from build123d import *

# Parameters (mm, degrees)
BOSS_EXTRUDE2_DEPTH = 12
SKETCH2_W           = 12
SKETCH2_H           = 22.5
BOSS_EXTRUDE3_DEPTH = 6
SKETCH3_W           = 12
SKETCH3_H           = 22.5
BOSS_EXTRUDE4_DEPTH = 6
SKETCH4_R           = 1.75
CUT_EXTRUDE1_DEPTH  = 22.5
FILLET1_R           = 2
BOSS_EXTRUDE5_START = 4.65
BOSS_EXTRUDE5_DEPTH = 4.65
SKETCH6_W           = 26.4
SKETCH6_H           = 18
SKETCH6_R           = 4.925
BOSS_EXTRUDE6_DEPTH = 2.5


with BuildPart() as part:
    # Sketch1 → Boss-Extrude2 (new body)
    with BuildSketch(Plane.XY):
        Polygon((0, 18), (0, 0), (17.3, 0), (17.3, 7.6), (17.3, 15.2), (20.697059459, 15.2), (34.302940541, 15.2), (37.7, 15.2), (37.7, 7.6), (37.7, 0), (55, 0), (55, 18), align=None)
        with BuildLine():
            Line((17.3, 15.2), (17.3, 7.6))
            ThreePointArc((17.3, 7.6), (18.187911257, 11.762331467), (20.697059459, 15.2))
            Line((20.697059459, 15.2), (17.3, 15.2))
        make_face()
        with BuildLine():
            Line((37.7, 15.2), (34.302940541, 15.2))
            ThreePointArc((34.302940541, 15.2), (36.812088743, 11.762331467), (37.7, 7.6))
            Line((37.7, 7.6), (37.7, 15.2))
        make_face()
    extrude(amount=BOSS_EXTRUDE2_DEPTH)

    # Sketch2 → Boss-Extrude3 (add)
    with BuildSketch(Plane.ZY):
        with Locations((6, 6.75)):
            Rectangle(SKETCH2_W, SKETCH2_H)
    extrude(amount=BOSS_EXTRUDE3_DEPTH)

    # Sketch3 → Boss-Extrude4 (add)
    with BuildSketch(Plane(origin=(55, 0, 0), x_dir=(0, 0, -1), z_dir=(1, 0, 0))):
        with Locations((-6, 6.75)):
            Rectangle(SKETCH3_W, SKETCH3_H)
    extrude(amount=BOSS_EXTRUDE4_DEPTH)

    # Sketch4 → Cut-Extrude1 (cut)
    with BuildSketch(Plane(origin=(0, 18, 0), x_dir=(1, 0, 0), z_dir=(0, 1, 0))):
        with Locations(Location((-3, -7, 0), (0, 0, 270))):
            Circle(SKETCH4_R)
        with Locations(Location((58, -7, 0), (0, 0, 270))):
            Circle(SKETCH4_R)
    extrude(amount=-CUT_EXTRUDE1_DEPTH, mode=Mode.SUBTRACT)

    # Fillet1
    # the kernel refuses this fillet: 2 mm, written as the material it takes off along each edge
    with BuildSketch(Plane(origin=(-3, 18, 7), x_dir=(0, 0, 1), z_dir=(-1, 0, 0))) as fillet1_piece_1:
        with BuildLine():
            CenterArc((1.75 + FILLET1_R, -FILLET1_R), FILLET1_R, 90, 90)
            Line((1.75, -FILLET1_R), (1.75, 0))
            Line((1.75, 0), (1.75 + FILLET1_R, 0))
        make_face()
    revolve(axis=Axis((-3, 18, 7), (0, 1, 0)), mode=Mode.SUBTRACT)
    with BuildSketch(Plane(origin=(58, 18, 7), x_dir=(0, 0, 1), z_dir=(-1, 0, 0))) as fillet1_piece_2:
        with BuildLine():
            CenterArc((1.75 + FILLET1_R, -FILLET1_R), FILLET1_R, 90, 90)
            Line((1.75, -FILLET1_R), (1.75, 0))
            Line((1.75, 0), (1.75 + FILLET1_R, 0))
        make_face()
    revolve(axis=Axis((58, 18, 7), (0, 1, 0)), mode=Mode.SUBTRACT)

    # Sketch5 → Boss-Extrude5 (add)
    with BuildSketch(Plane(origin=(0, 0, 0), x_dir=(-1, 0, 0), z_dir=(0, 0, -1)).offset(BOSS_EXTRUDE5_START)):
        with BuildLine():
            Line((-37.7, 0), (-40.7, 0))
            Line((-40.7, 0), (-40.7, 18))
            Line((-40.7, 18), (-14.3, 18))
            Line((-14.3, 18), (-14.3, 0))
            Line((-14.3, 0), (-17.3, 0))
            Line((-17.3, 0), (-17.3, 6))
            ThreePointArc((-17.3, 6), (-18.898767331, 7.537206525), (-17.425490196, 9.195071224))
            ThreePointArc((-17.425490196, 9.195071224), (-18.543054375, 12.47986937), (-20.697059459, 15.2))
            Line((-20.697059459, 15.2), (-34.302940541, 15.2))
            ThreePointArc((-34.302940541, 15.2), (-36.456945625, 12.47986937), (-37.574509804, 9.195071224))
            ThreePointArc((-37.574509804, 9.195071224), (-36.101232669, 7.537206525), (-37.7, 6))
            Line((-37.7, 6), (-37.7, 0))
        make_face()
    extrude(amount=-BOSS_EXTRUDE5_DEPTH)

    # Sketch6 → Boss-Extrude6 (add)
    with BuildSketch(Plane(origin=(0, 0, -4.65), x_dir=(-1, 0, 0), z_dir=(0, 0, -1))):
        with Locations((-27.5, 9)):
            Rectangle(SKETCH6_W, SKETCH6_H)
        with Locations((-27.5, 7.537206525)):
            Circle(SKETCH6_R, mode=Mode.SUBTRACT)
    extrude(amount=BOSS_EXTRUDE6_DEPTH)


solid = part.part
Verification items for the finished model (mm, model axes). A direction names the side the tool comes from. Give positions to 0.01 mm unless a question says otherwise; leave off trailing zeros. Order: outer loops, then holes, each group sorted by start corner. A loop starts at its lowest first (then second) coordinate and runs counter-clockwise, first axis right, second up. Notation, with made-up numbers: M 13,32.5 L 25,32.5 A15 ccw 25,61.5 Z; hole C 28.5,57 d10. An arc over 180 degrees is marked long. Use one line per item in the form item = value. Start each with the question number.
Q1. Mould release check, pull along Y, two halves, no side actions. Record for faces 1 (the cylindrical face through (36.1, 7.6, -2.4)), 2 (the flat face through (55, -2, 6)), 3 (the flat face through (28, 18, 5)), 4 (the cylindrical face through (31.41, 4.54, -5.88)): +Y half, -Y half, draft (parallel to the pull), parting line (faces both ways), or undercut.
Q2. Scan lines: line 1 along X through (y, z) = (2.5, 7); line 2 along X through (y, z) = (-1.5, 1.5); line 3 along Y through (x, z) = (27.5, -5.7). Record each from-to range of solid material in increasing order. Write a range as [from, to].
Q3. Section check B-B (y = 1.5). Enter the section's corners in (x, z).
Q4. Go/stop test with flat-tipped pins: pin 1 Ø8 at (x, y) = (27, -0.5) entering from +Z; pin 2 Ø6 at (x, y) = (7, 6.5) entering from -Z; pin 3 Ø1 at (y, z) = (5.5, -1) entering from +X. Record where each tip stops, or that it passes through.
Q5. Section check C-C (z = 7). Enter the section's corners in (x, y), then the cut area to 3 significant figures.
Q6. Section check A-A (x = -3). Enter the section's corners in (y, z).
Q7. Section check D-D (y = 11.5). Enter the section's corners in (x, z).
Q8. Access from +Z, -Z, +X, -X, +Y, -Y to the whole of each face (thin tool, end or side, straight path). Record for faces 5 (the flat face through (51, 9, 0)), 6 (the flat face through (17.3, 4, 4)), 7 (the flat face through (28, 0, -6)).
Evaluation:
q1.face_1 = undercut
q1.face_2 = draft
q1.face_3 = +Y half
q1.face_4 = undercut
q2.line_1 = [-6, -4.75], [-1.25, 17.3], [37.7, 56.25], [59.75, 61]
q2.line_2 = [-6, 0], [55, 61]
q2.line_3 = [0, 2.61], [12.46, 18]
q3.outline = M -6,0 L 14.3,0 L 14.3,-7.15 L 40.7,-7.15 L 40.7,0 L 61,0 L 61,12 L 37.7,12 L 37.7,-4.65 L 17.3,-4.65 L 17.3,12 L -6,12 Z; hole C -3,7 d3.5; hole C 58,7 d3.5
q4.pin_1 = -4.65
q4.pin_2 = 0
q4.pin_3 = 40.7
q5.outline = M -6,-4.5 L -4.75,-4.5 L -4.75,16 A2 ccw -6,17.85 Z; M -1.25,-4.5 L 0,-4.5 L 0,0 L 17.3,0 L 17.3,7.6 A10.2 cw 20.7,15.2 L 34.3,15.2 A10.2 cw 37.7,7.6 L 37.7,0 L 55,0 L 55,-4.5 L 56.25,-4.5 L 56.25,16 A2 ccw 54.25,18 L 0.75,18 A2 ccw -1.25,16 Z; M 59.75,-4.5 L 61,-4.5 L 61,17.85 A2 ccw 59.75,16 Z
q5.area = 805 mm2
q6.outline = M -4.5,0 L 18,0 L 18,3.25 A2 ccw 16,5.25 L -4.5,5.25 Z; M -4.5,8.75 L 16,8.75 A2 ccw 18,10.75 L 18,12 L -4.5,12 Z
q7.outline = M -6,0 L 14.3,0 L 14.3,-7.15 L 24.58,-7.15 L 24.58,-4.65 L 18.08,-4.65 L 18.08,12 L -6,12 Z; M 30.42,-7.15 L 40.7,-7.15 L 40.7,0 L 61,0 L 61,12 L 36.92,12 L 36.92,-4.65 L 30.42,-4.65 Z; hole C -3,7 d3.5; hole C 58,7 d3.5
q8.face_5 = -Z, +X, +Y, -Y
q8.face_6 = +Z, -Y
q8.face_7 = +Z, -Z, -Y
